Autodesk Inventor part; units mm, degrees
ref_plane "YZ Plane" through (0, 0, 0) normal (1, 0, 0) x (0, 1, 0)
ref_plane "XZ Plane" through (0, 0, 0) normal (0, 1, 0) x (-1, 0, 0)
ref_plane "XY Plane" through (0, 0, 0) normal (0, 0, 1) x (1, 0, 0)
sketch "Sketch1" plane through (0, 0, 0) normal (0, 0, 1) x (1, 0, 0)
  line L0 (-15, -15) -> (-15, 15)
  line L1 (-15, 15) -> (15, 15)
  line L2 (15, 15) -> (15, -15)
  line L3 (15, -15) -> (-15, 15) construction
  line L4 (-15, -15) -> (15, 15) construction
  line L5 (0, 0) -> (8.0802, 0) construction
  line L6 (0, 0) -> (0, 7.2946) construction
  line L7 (-5.05, -20.05) -> (5.05, -20.05)
  line L8 (5.05, -20.05) -> (5.05, -6.05)
  line L9 (5.05, -6.05) -> (-5.05, -6.05)
  line L10 (-5.05, -6.05) -> (-5.05, -20.05)
  line L11 (-5.05, -20.05) -> (5.05, -6.05) construction
  line L12 (5.05, -20.05) -> (-5.05, -6.05) construction
  line L13 (15, -15) -> (5.05, -15)
  line L14 (-5.05, -15) -> (-15, -15)
  point P0 (-12, -12.5)
  point P1 (12, -12.5)
  point P2 (-12, 12.5)
  point P3 (12, 12.5)
  point P4 (0, -13.05)
  dimension "d0" = 30
  dimension "d1" = 30
  dimension "d4" = 24
  dimension "d7" = 25
  dimension "d10" = 10.1
  dimension "d11" = 14
extrude "Extrusion1" add sketch "Sketch1" along normal blind 15 contours L0 L1 L2 L13 L8 L9 L10 L14
hole "Hole1" at (12, 12.5, 0) at (-12, 12.5, 0) at (-12, -12.5, 0) at (12, -12.5, 0) direction (0, 0, 1) diameter 2.9 end through all
sketch "Sketch2" plane through (0, 0, 0) normal (0, 0, -1) x (-1, 0, 0)
  point P0 (0, 0)
  point P1 (0, 0)
hole "Hole2" at (0, 0, 0) direction (0, 0, 1) diameter 5.3 end through all
sketch "Sketch3" plane through (0, 0, 15) normal (0, 0, 1) x (1, 0, 0)
  line L0 (15, 15) -> (-15, 15)
  line L1 (-15, 15) -> (-9, 15)
  line L2 (-9, 15) -> (-9, 10)
  line L3 (-9, 10) -> (-15, 10)
  line L4 (-15, 10) -> (-15, 15)
  line L5 (15, -15) -> (15, 15)
  line L6 (15, 15) -> (9, 15)
  line L7 (9, 15) -> (9, 10)
  line L8 (9, 10) -> (15, 10)
  line L9 (15, 10) -> (15, 15)
  line L10 (-15, -15) -> (-5.05, -15)
  line L11 (-15, -15) -> (-9, -15)
  line L12 (-9, -15) -> (-9, -10)
  line L13 (-9, -10) -> (-15, -10)
  line L14 (-15, -10) -> (-15, -15)
  line L15 (15, -15) -> (9, -15)
  line L16 (9, -15) -> (9, -10)
  line L17 (9, -10) -> (15, -10)
  line L18 (15, -10) -> (15, -15)
  circle A0 centre (0, 0) radius 2.65
  circle A1 centre (-12, -12.5) radius 1.45
  circle A2 centre (12, 12.5) radius 1.45
  circle A3 centre (-12, 12.5) radius 1.45
  circle A4 centre (12, -12.5) radius 1.45
  line L19 (15, 15) -> (-15, 15)
  line L20 (-15, 15) -> (-15, -15)
  line L21 (-15, -15) -> (-5.05, -15)
  line L22 (-5.05, -15) -> (-5.05, -6.05)
  line L23 (-5.05, -6.05) -> (5.05, -6.05)
  line L24 (5.05, -6.05) -> (5.05, -15)
  line L25 (5.05, -15) -> (15, -15)
  line L26 (15, -15) -> (15, 15)
  dimension "d28" = 6
  dimension "d29" = 5
  dimension "d30" = 6
  dimension "d31" = 5
  dimension "d32" = 6
  dimension "d33" = 5
extrude "Extrusion2" cut sketch "Sketch3" against normal blind 2 contours L7 L8 L5 L17 L16 L25 L24 L23 L22 L10 L12 L13 L20 L3 L2 L0
sketch "Sketch4" plane through (0, 0, 13) normal (0, 0, 1) x (1, 0, 0)
  line L0 (2.3671, 4.1) -> (4.7343, 0)
  line L1 (4.7343, 0) -> (2.3671, -4.1)
  line L2 (2.3671, -4.1) -> (-2.3671, -4.1)
  line L3 (-2.3671, -4.1) -> (-4.7343, 0)
  line L4 (-4.7343, 0) -> (-2.3671, 4.1)
  line L5 (-2.3671, 4.1) -> (2.3671, 4.1)
  point P0 (0, 0)
  point P1 (0, 0)
  dimension "d36" = 8.2
extrude "Extrusion3" cut sketch "Sketch4" against normal blind 10
properties part number "front_door-webcam(FIT0701)-mount"
Verification items for the finished model (mm, model axes). A direction names the side the tool comes from. Give positions to 0.01 mm unless a question says otherwise; leave off trailing zeros. Order: outer loops, then holes, each group sorted by start corner. A loop starts at its lowest first (then second) coordinate and runs counter-clockwise, first axis right, second up. Notation, with made-up numbers: M 1,-29.75 L 57,-29.75 A26 ccw 57,-7.75 Z; hole C 70,84 d4. An arc over 180 degrees is marked long. Return JSON: item names as keys, results as strings. Group by question number.
1) Section check A-A on z = 12.25. Record the cut outline in (x, y).
2) Section check D-D on y = 2. Record the cut outline in (x, z), and give its area (3 significant figures).
3) Section check C-C on x = 0. Record the cut outline in (y, z), and give its area (3 significant figures).
4) Mould release check, pull along X, two halves, no side actions. Record for faces 4 (the face through (-10, -15, 7)), 5 (the face through (-9, -13, 14)): pulls with the +X half, pulls with the -X half, needs draft (parallel to the pull), parting line crosses it, or undercut.
5) Scan lines: line 1 (Y direction, x = 12, z = 7); line 2 (X direction, y = 12.5, z = 5.75); line 3 (Y direction, x = -12, z = 13.5). Record each from-to range of solid material in increasing order.
6) Section check B-B on y = 12.5. Record the cut outline in (x, z).
7) Access from +Z, -Z, +X, -X, +Y, -Y to the whole of each face (thin tool, end or side, straight path). Record for faces 1 (the face through (-12, -10, 14)), 2 (the face through (9, 13, 14)), 3 (the face through (3.534, 2.079, 8.07)).
8) Go/stop test with flat-tipped pins: pin 1 Ø8 at (x, y) = (2.5, -3) entering from +Z; pin 2 Ø2 at (x, z) = (0.5, 3.5) entering from -Y; pin 3 Ø1.7 at (x, y) = (12, -12.5) entering from -Z; pin 4 Ø4 at (x, y) = (-0.5, -1) entering from +Z. Record where each tip stops, or that it passes through.
Answer block:
{
 "1": {"outline": "M -15,-15 L -5.05,-15 L -5.05,-6.05 L 5.05,-6.05 L 5.05,-15 L 15,-15 L 15,15 L -15,15 Z; hole C -12,-12.5 d2.9; hole C -12,12.5 d2.9; hole M -4.73,0 L -2.37,-4.1 L 2.37,-4.1 L 4.73,0 L 2.37,4.1 L -2.37,4.1 Z; hole C 12,-12.5 d2.9; hole C 12,12.5 d2.9"},
 "2": {"outline": "M -15,0 L -1.74,0 L -1.74,3 L -3.58,3 L -3.58,13 L -15,13 Z; M 1.74,0 L 15,0 L 15,13 L 3.58,13 L 3.58,3 L 1.74,3 Z", "area": "308 mm^2"},
 "3": {"outline": "M -6.05,0 L -2.65,0 L -2.65,3 L -4.1,3 L -4.1,13 L -6.05,13 Z; M 2.65,0 L 15,0 L 15,13 L 4.1,13 L 4.1,3 L 2.65,3 Z", "area": "176 mm^2"},
 "4": {"face 4": "needs draft", "face 5": "undercut"},
 "5": {"line 1": "y = -15 to -13.95, -11.05 to 11.05, 13.95 to 15", "line 2": "x = -15 to -13.45, -10.55 to 10.55, 13.45 to 15", "line 3": "y = -15 to -13.95, -11.05 to -10, 10 to 11.05, 13.95 to 15"},
 "6": {"outline": "M -15,0 L -13.45,0 L -13.45,15 L -15,15 Z; M -10.55,0 L 10.55,0 L 10.55,15 L 9,15 L 9,13 L -9,13 L -9,15 L -10.55,15 Z; M 13.45,0 L 15,0 L 15,15 L 13.45,15 Z"},
 "7": {"face 1": "+Z, +X, -X", "face 2": "+Z, +Y, -Y", "face 3": "+Z"},
 "8": {"pin 1": "stops at z = 13", "pin 2": "stops at y = -6.05", "pin 3": "passes through", "pin 4": "stops at z = 3"}
}
